```python
from build123d import *

# Parameters (mm, degrees)
F3_DEPTH = 4
F6_SIZE  = 0.5


with BuildPart() as f1:
    # F0 (on Front) → F1 (revolve)
    with BuildSketch(Plane.XZ):
        Polygon((0, 20.3999999762), (0, 0), (2.5, 0), (2.5, 20), (4, 20), (4, 20.3999999762), align=None)
    revolve(axis=Axis((0, 0, 10.1999999881), (0, 0, 1)))

    # F2 (on face) → F3 (join)
    with BuildSketch(Plane.XY.offset(20.3999999762)):
        with BuildLine():
            ThreePointArc((2.249999971, -3.8971143338), (3.8971143086, -2.2500000145), (4.5, 0))
            ThreePointArc((4.5, 0), (3.8971143176, 2.249999999), (2.250000002, 3.8971143159))
            ThreePointArc((2.250000002, 3.8971143159), (-2.9e-08, 4.5), (-2.2500000522, 3.8971142869))
            ThreePointArc((-2.2500000522, 3.8971142869), (-3.8971143321, 2.2499999739), (-4.5, 0))
            ThreePointArc((-4.5, 0), (-3.8971143245, -2.2499999871), (-2.2500000257, -3.8971143022))
            ThreePointArc((-2.2500000257, -3.8971143022), (-3.16e-08, -4.5), (2.249999971, -3.8971143338))
        make_face()
        with BuildLine():
            Line((4.5, -2.5980762114), (4.5, 0))
            ThreePointArc((4.5, 0), (3.8971143086, -2.2500000145), (2.249999971, -3.8971143338))
            Line((2.249999971, -3.8971143338), (4.5, -2.5980762114))
        make_face()
        with BuildLine():
            ThreePointArc((2.250000002, 3.8971143159), (3.8971143176, 2.249999999), (4.5, 0))
            Line((4.5, 0), (4.5, 2.5980762114))
            Line((4.5, 2.5980762114), (2.250000002, 3.8971143159))
        make_face()
        with BuildLine():
            ThreePointArc((-2.2500000522, 3.8971142869), (-2.9e-08, 4.5), (2.250000002, 3.8971143159))
            Line((2.250000002, 3.8971143159), (0, 5.1961524227))
            Line((0, 5.1961524227), (-2.2500000522, 3.8971142869))
        make_face()
        with BuildLine():
            Line((0, -5.1961524227), (2.249999971, -3.8971143338))
            ThreePointArc((2.249999971, -3.8971143338), (-3.16e-08, -4.5), (-2.2500000257, -3.8971143022))
            Line((-2.2500000257, -3.8971143022), (0, -5.1961524227))
        make_face()
        with BuildLine():
            ThreePointArc((-4.5, 0), (-3.8971143321, 2.2499999739), (-2.2500000522, 3.8971142869))
            Line((-2.2500000522, 3.8971142869), (-4.5, 2.5980762114))
            Line((-4.5, 2.5980762114), (-4.5, 0))
        make_face()
        with BuildLine():
            Line((-4.5, -2.5980762114), (-2.2500000257, -3.8971143022))
            ThreePointArc((-2.2500000257, -3.8971143022), (-3.8971143245, -2.2499999871), (-4.5, 0))
            Line((-4.5, 0), (-4.5, -2.5980762114))
        make_face()
    extrude(amount=F3_DEPTH)

    # F4 (on Front) → F5 (revolve, cut)
    with BuildSketch(Plane.XZ):
        Polygon((-7.9641016151, 22.3999999762), (-4.5, 24.3999999762), (-9.8750129299, 24.3999999762), (-9.8750129299, 23.5032651381), align=None)
        Polygon((-4.5, 20.3999999762), (-7.9641016151, 22.3999999762), (-9.8750129299, 21.2967348142), (-9.8750129299, 20.3999999762), align=None)
        Polygon((-9.8750129299, 21.2967348142), (-7.9641016151, 22.3999999762), (-9.8750129299, 23.5032651381), align=None)
    revolve(axis=Axis((0, 0, 22.3999999762), (0, 0, -1)), mode=Mode.SUBTRACT)

    # F6
    f6_edges = [f1.edges().sort_by_distance(p)[0] for p in [
        (-2.5, 0, 0),
    ]]
    chamfer(f6_edges, length=F6_SIZE)


solid = f1.part
```
Source: CAD feature listing. Evaluate the final solid. Frame: model axes, mm. A direction names the side the tool comes from. Round coordinates to 2 decimals unless told otherwise and drop trailing zeros. Loops run counter-clockwise (first coordinate to the right, second up) from the corner with the lowest first, then second, coordinate; pieces in that order, holes last. Notation, with made-up numbers: M 77,32.5 L 110,32.5 A25 cw 110,62.5 Z; hole C 42.5,-1.5 d3. An arc over 180 degrees is marked long. Use a Markdown table: item, result. Add a question column.
1. Contact query for flat-ended pins moving along their axis: pin 1 (4 mm diameter, centred on y = -1, z = 5, fed in from +X); pin 2 (1 mm diameter, centred on x = 1.5, z = 8, fed in from -Y); pin 3 (1.5 mm diameter, centred on y = 2.5, z = 19, fed in from -X). Output: stop coordinate, or through.
2. Ray query, line 1 along Z through (x, y) = (-1.25, 2.5); line 2 along Z through (x, y) = (1, 4.25); line 3 along X through (y, z) = (1.5, 15.5). Return the intervals inside material, ascending. Write a range as [from, to].
3. Cut plane A-A, the plane z = 9.75. Output: boundary loops of the cut face in (x, y).
4. Set-up query: faces 1 (the cylindrical face through (-0.54, -2.44, 10.39)), 2 (the conical face through (4.049, -2.325, 20.498)). Return all of +Z, -Z, +X, -X, +Y, -Y with unobstructed straight access to the full face (end or side cutting, diameter ignored); none if empty.
Solution:
| question | item | result |
|---|---|---|
| 1 | pin 1 | stops at x = 2.5 |
| 1 | pin 2 | stops at y = -2.29 |
| 1 | pin 3 | stops at x = -1.79 |
| 2 | line 1 | z = [20, 24.4] |
| 2 | line 2 | z = [20.4, 24.4] |
| 2 | line 3 | x = [-2, 2] |
| 3 | outline | C 0,0 d5 |
| 4 | face 1 | -Z |
| 4 | face 2 | -Z, +X, -Y |
